Could you check a few things on this model? Use its own coordinates, in mm. A direction names the side the tool comes from. Give positions to 0.01 mm unless a question says otherwise; leave off trailing zeros. Loops run counter-clockwise (first coordinate to the right, second up) from the corner with the lowest first, then second, coordinate; pieces in that order, holes last. Notation, with made-up numbers: (52.5, 56.5) - (85.5, 56.5) arc R14 cw to (85.5, 68.5) - close; hole circle Ø5 at (64, -14.75). An arc over 180 degrees is marked (long way). Write each question's results on one line, items separated by ' | '. Start each with the question number.
(1) If we mould it in two halves opening along Z, with no side actions, what happens to faces 4 (the face through (2.465, 43.171, 16.743)), 5 (the face through (2, 41, 87.864)), 6 (the face through (2, 13, 50.599))? For each: released by +Z, released by -Z, zero draft, split by the parting line, or undercut.
(2) I need wall thicknesses on line 1 (Z direction, x = 1.9, y = 74.5); line 2 (Z direction, x = 4.3, y = 11); line 3 (Y direction, x = 2.6, z = 38.5). Which ranges of each line are inside material? Lowest first, please.
(3) For pin 1 (2.5 mm diameter, centred on x = 2, y = 14.5, fed in from -Z); pin 2 (2.5 mm diameter, centred on x = 1.5, y = 57.5, fed in from -Z); pin 3 (2.5 mm diameter, centred on x = 3.5, z = -5.5, fed in from +Y), each with a flat end and sliding along its axis, tell me the tip position at first contact or that it passes through.
(4) Suppose I cut it at C-C (y = 48.5). Please give me the cut outline in (x, z), and give its area (3 significant figures).
(5) On a 3-axis mill with a long thin cutter (end or side, diameter ignored), from which of +Z, -Z, +X, -X, +Y, -Y can I reach the whole of each face in a straight line? I mean faces 1 (the face through (2, 21.458, 22)), 2 (the face through (2, 34.458, -4)), 3 (the face through (3, 78.369, 43)). Say none if no direction works.
(6) Suppose I cut it at A-A (x = 1.9). Please give me the cut outline in (y, z).
(7) Suppose I cut it at B-B (z = 5). Please give me the cut outline in (x, y), and give its area (3 significant figures).
Solid Edge part; units mm, degrees
sketch "Sketch1" plane through (0, 0, 0) normal (1, 0, 0) x (0, 1, 0)
  line L0 (21.4576, 50.5988) -> (21.4576, -7.2012)
  line L1 (34.4576, -7.2012) -> (21.4576, -7.2012)
  line L2 (34.4576, 50.5988) -> (34.4576, -7.2012)
  line L3 (34.4576, 50.5988) -> (21.4576, 50.5988)
extrude "Protrusion1" add sketch "Sketch1" along normal blind 5
sketch "Sketch2" plane through (2.5, 26.4576, 50.5988) normal (0, 0, 1) x (0, 1, 0)
  line L0 (-5, -2.5) -> (5, -2.5)
  line L1 (5, -2.5) -> (5, 2.5)
  line L2 (5, 2.5) -> (-5, 2.5)
  line L3 (-48.6449, 2.5) -> (-5, 2.5)
  line L4 (-48.6449, -2.5) -> (-48.6449, 2.5)
  line L5 (-5, -2.5) -> (-48.6449, -2.5)
extrude "ExtrudedProtrusion_2" add sketch "Sketch2" along normal blind 37.265
sketch "Sketch3" plane through (2.5, 31.4576, 40.3313) normal (0, 1, 0) x (0, 0, -1)
  line L0 (40.3303, 2.5) -> (-47.5325, 2.5)
  line L1 (-47.5325, -2.5) -> (-47.5325, 2.5)
  line L2 (40.3303, -2.5) -> (-47.5325, -2.5)
  line L3 (40.3303, -2.5) -> (40.3303, 2.5)
extrude "ExtrudedProtrusion_3" add sketch "Sketch3" along normal blind 46.9115
sketch "Sketch4" plane through (2.5, 28.0909, 87.8638) normal (0, 0, 1) x (0, 1, 0)
  line L0 (-24.7782, 2.5) -> (-24.7782, -2.5)
  line L1 (-24.7782, -2.5) -> (-51.7696, -2.5)
  line L2 (-51.7696, -2.5) -> (-51.7696, 2.5)
  line L3 (-51.7696, 2.5) -> (-24.7782, 2.5)
extrude "ExtrudedCutout_2" cut sketch "Sketch4" against normal blind 243.9976
sketch "Sketch5" plane through (0, 40.8409, 40.3313) normal (-1, 0, 0) x (0, 0, -1)
  circle A0 centre (23.9675, -0.6222) radius 1.75
extrude "ExtrudedCutout_3" cut sketch "Sketch5" against normal blind 61.0187
Output values:
1) face 4: undercut | face 5: released by +Z | face 6: released by -Z
2) line 1: 0 to 87.86 | line 2: 50.6 to 87.86 | line 3: 21.46 to 78.37
3) pin 1: z = 50.6 | pin 2: z = 0 | pin 3: y = 34.46
4) outline: (0, 0) - (5, 0) - (5, 87.86) - (0, 87.86) - close | area: 439 mm2
5) face 1: -Z, +X, -X, -Y | face 2: -Z, +X, -X, +Y | face 3: +Z, -Z, +X, -X, +Y
6) outline: (3.31, 50.6) - (21.46, 50.6) - (21.46, -7.2) - (34.46, -7.2) - (34.46, 0) - (78.37, 0) - (78.37, 87.86) - (3.31, 87.86) - close; hole circle Ø3.5 at (41.46, 16.36)
7) outline: (0, 21.46) - (5, 21.46) - (5, 78.37) - (0, 78.37) - close | area: 285 mm2
